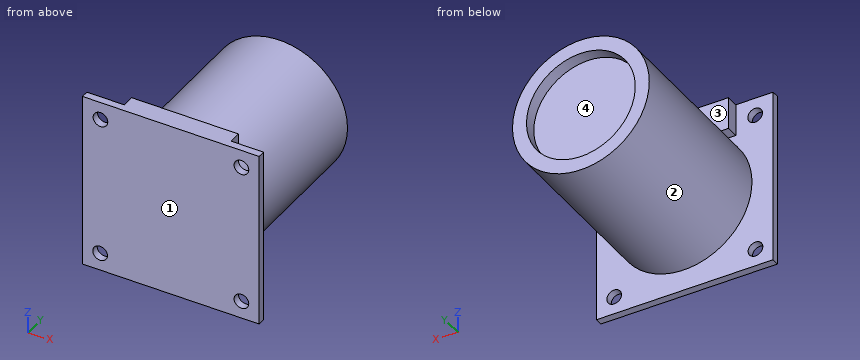
Autodesk Inventor part; units mm, degrees
ref_plane "YZ Plane" through (0, 0, 0) normal (1, 0, 0) x (0, 1, 0)
ref_plane "XZ Plane" through (0, 0, 0) normal (0, 1, 0) x (-1, 0, 0)
ref_plane "XY Plane" through (0, 0, 0) normal (0, 0, 1) x (1, 0, 0)
sketch "Sketch1" plane through (0, 0, 0) normal (0, 1, 0) x (-1, 0, 0)
  line L0 (0, 0) -> (36.068, 0)
  line L1 (36.068, 0) -> (36.068, -36.068)
  line L2 (36.068, -36.068) -> (0, -36.068)
  line L3 (0, -36.068) -> (0, 0)
  dimension "d0" = 36.068
  dimension "d1" = 36.068
extrude "Extrusion1" add sketch "Sketch1" along normal blind 1.524
sketch "Sketch2" plane through (0, 1.524, 0) normal (0, 1, 0) x (1, 0, 0)
  circle A0 centre (-17.78, 17.78) radius 13.97
  line L0 (0, 0) -> (0, 36.068)
  line L1 (-36.068, 0) -> (0, 0)
  dimension "d4" = 27.94
  dimension "d5" = 17.78
  dimension "d6" = 17.78
extrude "Extrusion2" add sketch "Sketch2" along normal blind 35.56
sketch "Sketch4" plane through (0, 1.524, 0) normal (0, 1, 0) x (1, 0, 0)
  line L0 (-28.448, 0) -> (-6.604, 0)
  line L1 (-6.604, 0) -> (-6.604, 6.604)
  line L2 (-6.604, 6.604) -> (-28.448, 6.604)
  line L3 (-28.448, 6.604) -> (-28.448, 0)
  line L4 (-36.068, 36.068) -> (-36.068, 0)
  point P0 (0, 0)
  dimension "d9" = 21.844
  dimension "d10" = 6.604
  dimension "d11" = 7.62
extrude "Extrusion3" add sketch "Sketch4" along normal blind 2.54
sketch "Sketch5" plane through (-17.78, 37.084, -17.78) normal (0, 1, 0) x (1, 0, 0)
  circle A0 centre (0, 0) radius 11.1186
  point P0 (17.78, -17.78)
extrude "Extrusion4" cut sketch "Sketch5" against normal blind 2.54
sketch "Sketch6" plane through (0, 1.524, 0) normal (0, 1, 0) x (1, 0, 0)
  circle A0 centre (-32.4, 3.6681) radius 1.5
  circle A1 centre (-32.468, 32.468) radius 1.5
  circle A2 centre (-3.6, 3.668) radius 1.5
  circle A3 centre (-3.6, 32.468) radius 1.5
  line L0 (0, 36.068) -> (-36.068, 36.068)
  line L1 (0, 0) -> (0, 36.068)
  line L2 (-36.068, 36.068) -> (-36.068, 0)
  dimension "d16" = 3
  dimension "d17" = 3
  dimension "d18" = 3
  dimension "d19" = 3
  dimension "d20" = 28.8
  dimension "d21" = 28.8
  dimension "d22" = 3.6
  dimension "d23" = 3.6
  dimension "d24" = 3.6
  dimension "d25" = 3.6
  dimension "d26" = 3.6
extrude "Extrusion5" cut sketch "Sketch6" against normal up to surface (1.524 mm away)
properties part number "camera"
Check sheet for the modelled part. Datum: model origin and axes. Units: mm. Face numbers are marked on the shaded views. A direction names the side the tool comes from. Give positions to 0.01 mm unless a question says otherwise; leave off trailing zeros. Write each loop counter-clockwise with the first axis right and the second up, starting at its lowest first coordinate (ties: lowest second). Pieces come first, ordered by that corner, then holes. Notation, with made-up numbers: (42.25, 74.25) -> (66.25, 74.25) arc R5 ccw to (66.25, 83.25) -> close; hole circle Ø10 at (35, 83). An arc over 180 degrees is marked (long way). Use CSV: the item, a comma, the result in double quotes. Start each with the question number.
Q1. Cross-section at C-C on x = -32.4. Enter the section's corners in (y, z), and give its area (3 significant figures).
Q2. Depth check by flat-ended pin: P1, Ø0.8, axis at y = 2.5, z = -2.5, coming from the -X side; P2, Ø0.8, axis at y = 2.5, z = -3, coming from the +X side; P3, Ø10, axis at x = -24, y = 7.5, coming from the -Z side. Enter the tip coordinate at first touch or a pass-through.
Q3. Cross-section at D-D on y = 25.5. Enter the section's corners in (x, z), and give its area (3 significant figures).
Q4. Scan lines: line 1 along Z through (x, y) = (-3.6, 0.9); line 2 along Z through (x, y) = (-17.78, 36.55); line 3 along Y through (x, z) = (-21, -13). Record each from-to range of solid material in increasing order.
Q5. Release check for a two-part mould opening along Z. For the marked faces 3 and 4 record: +Z half, -Z half, draft (parallel to the pull), parting line (faces both ways), or undercut.
Q6. Cross-section at A-A on z = -17.78. Enter the section's corners in (x, y).
Q7. Cross-section at B-B on x = -17.78. Enter the section's corners in (y, z).
Q8. Tool access check on the marked faces 1 and 2. Record the directions out of +Z, -Z, +X, -X, +Y, -Y that give a thin tool (end or side, any length) a straight path to the whole face; none if there is none.
Working result:
1,outline,"(0, -36.07) -> (1.52, -36.07) -> (1.52, -33.97) -> (0, -33.97) -> close; (0, -30.97) -> (1.52, -30.97) -> (1.52, -5.17) -> (0, -5.17) -> close; (0, -2.17) -> (1.52, -2.17) -> (1.52, 0) -> (0, 0) -> close"
1,area,"45.8 mm^2"
2,P1,"stops at x = -28.45"
2,P2,"stops at x = -6.6"
2,P3,"stops at z = -31.7"
3,outline,"circle Ø27.94 at (-17.78, -17.78)"
3,area,"613 mm^2"
4,line 1,"z = -36.07 to -33.97, -30.97 to -5.17, -2.17 to 0"
4,line 2,"z = -31.75 to -28.9, -6.66 to -3.81"
4,line 3,"y = 0 to 34.54"
5,face 3,"draft"
5,face 4,"undercut"
6,outline,"(-36.07, 0) -> (0, 0) -> (0, 1.52) -> (-3.81, 1.52) -> (-3.81, 37.08) -> (-6.66, 37.08) -> (-6.66, 34.54) -> (-28.9, 34.54) -> (-28.9, 37.08) -> (-31.75, 37.08) -> (-31.75, 1.52) -> (-36.07, 1.52) -> close"
7,outline,"(0, -36.07) -> (1.52, -36.07) -> (1.52, -31.75) -> (37.08, -31.75) -> (37.08, -28.9) -> (34.54, -28.9) -> (34.54, -6.66) -> (37.08, -6.66) -> (37.08, -3.81) -> (4.06, -3.81) -> (4.06, 0) -> (0, 0) -> close"
8,face 1,"+Z, -Z, +X, -X, -Y"
8,face 2,"+Y"
